Build history of the part. All positions in model axes, mm. A direction names the side the tool comes from. Round coordinates to 2 decimals unless told otherwise and drop trailing zeros. Loops run counter-clockwise (first coordinate to the right, second up) from the corner with the lowest first, then second, coordinate; pieces in that order, holes last.
from build123d import *

# Parameters (mm, degrees)
SKETCH_R        = 3.6
SKETCH_R_2      = 2.6
PAD_DEPTH       = 18
SKETCH001_R     = 3.6
POCKET_DEPTH    = 3
SKETCH002_W     = 40
SKETCH002_H     = 100
POCKET001_DEPTH = 8
SKETCH003_R     = 5.5
SKETCH003_R_2   = 4.5
POCKET002_DEPTH = 6
FILLET_R        = 6
FILLET001_R     = 6
SKETCH004_W     = 6.5
SKETCH004_H     = 33
POCKET003_DEPTH = 4
SKETCH005_R     = 2.1
POCKET004_DEPTH = 10
FILLET002_R     = 3.75


with BuildPart() as part:
    # Sketch → Pad (new body)
    with BuildSketch(Plane.XY):
        Polygon((-38.5, 0), (-38.5, 10), (19, 40), (38.5, 40), (38.5, 0), (38.5, -40), (19, -40), (-38.5, -10), align=None)
        with Locations((-28.5, 0)):
            Circle(SKETCH_R, mode=Mode.SUBTRACT)
        with Locations((28.5, -30)):
            Circle(SKETCH_R_2, mode=Mode.SUBTRACT)
        with Locations((28.5, 30)):
            Circle(SKETCH_R_2, mode=Mode.SUBTRACT)
    extrude(amount=PAD_DEPTH)

    # Sketch001 (on Face3 of Pad) → Pocket (cut)
    with BuildSketch(Plane(origin=(0, 0, 0), x_dir=(1, 0, 0), z_dir=(0, 0, -1))):
        with Locations((-28.5, 0)):
            Circle(SKETCH001_R)
    extrude(amount=-POCKET_DEPTH, mode=Mode.SUBTRACT)

    # Sketch002 (on Face3 of Pocket) → Pocket001 (cut)
    with BuildSketch(Plane(origin=(0, 0, 0), x_dir=(1, 0, 0), z_dir=(0, 0, -1))):
        Rectangle(SKETCH002_W, SKETCH002_H)
    extrude(amount=-POCKET001_DEPTH, mode=Mode.SUBTRACT)

    # Sketch003 (on Face6 of Pocket001) → Pocket002 (cut)
    with BuildSketch(Plane.XY.offset(18)):
        with Locations((-28.5, 0)):
            Circle(SKETCH003_R)
        with Locations((28.5, 30)):
            Circle(SKETCH003_R_2)
        with Locations((28.5, -30)):
            Circle(SKETCH003_R_2)
    extrude(amount=-POCKET002_DEPTH, mode=Mode.SUBTRACT)

    # Fillet
    fillet_edges = [part.edges().sort_by_distance(p)[0] for p in [
        (20, -40, 4),
        (20, 40, 4),
        (-20, -19.652174, 4),
        (-20, 19.652174, 4),
    ]]
    fillet(fillet_edges, radius=FILLET_R)

    # Fillet001
    fillet001_edges = [part.edges().sort_by_distance(p)[0] for p in [
        (-38.5, 10, 9),
        (-38.5, -10, 9),
        (19, 40, 13),
        (38.5, 40, 9),
        (38.5, -40, 9),
        (19, -40, 13),
    ]]
    fillet(fillet001_edges, radius=FILLET001_R)

    # Sketch004 (on Face5 of Fillet001) → Pocket003 (cut)
    with BuildSketch(Plane.XY.offset(18)):
        with Locations((0, -18.5)):
            Rectangle(SKETCH004_W, SKETCH004_H)
        with Locations((0, 18.5)):
            Rectangle(SKETCH004_W, SKETCH004_H)
    extrude(amount=-POCKET003_DEPTH, mode=Mode.SUBTRACT)

    # Sketch005 (on Face6 of Pocket003) → Pocket004 (cut)
    with BuildSketch(Plane.XY.offset(18)):
        with Locations((-15, 0)):
            Circle(SKETCH005_R)
        with Locations((15, -30)):
            Circle(SKETCH005_R)
        with Locations((15, 30)):
            Circle(SKETCH005_R)
    extrude(amount=-POCKET004_DEPTH, mode=Mode.SUBTRACT)

    # Fillet002
    fillet002_edges = [part.edges().sort_by_distance(p)[0] for p in [
        (0, -2, 14),
        (0, 2, 14),
    ]]
    fillet(fillet002_edges, radius=FILLET002_R)


solid = part.part
(1) Slice it at B-B on x = 28.5. List the corners of the cut face in (y, z), plus the area to 3 significant figures.
Responses:
outline: (-40, 0) - (-32.6, 0) - (-32.6, 12) - (-34.5, 12) - (-34.5, 18) - (-40, 18) - close; (-27.4, 0) - (27.4, 0) - (27.4, 12) - (25.5, 12) - (25.5, 18) - (-25.5, 18) - (-25.5, 12) - (-27.4, 12) - close; (32.6, 0) - (40, 0) - (40, 18) - (34.5, 18) - (34.5, 12) - (32.6, 12) - close
area: 1,210 mm2
(2) Pull direction X, two halves, no side cores. Call faces 1 (the face through (-9.16, 25.31, 12.87)), 2 (the face through (36.789, 38.196, 9.126)), 3 (the face through (0, 19, 14)): +X half, -X half, draft (parallel to the pull), parting line (faces both ways), or undercut.
Responses:
face 1: -X half
face 2: +X half
face 3: undercut
(3) Which spindle directions (+Z, -Z, +X, -X, +Y, -Y) get a long thin tool onto all of the face, cutting with end or side? Do faces 4 (the face through (-3.25, -15, 16)), 5 (the face through (20, 0, 4)), 6 (the face through (-27, -4, 12)), 7 (the face through (-22.964, 14.929, 3.944)), 8 (the face through (-3.25, 15, 16)). Say none if no direction does.
Responses:
face 4: +Z, -Y
face 5: -Z, +Y, -Y
face 6: +Z
face 7: -Z, +Y
face 8: +Z, +Y
(4) Slice it at A-A on z = 5. List the corners of the cut face in (x, y).
Responses:
outline: (-38.5, -6.36) arc R6 ccw to (-35.28, -11.68) - (-28.78, -15.07) arc R6 ccw to (-20, -9.75) - (-20, 9.75) arc R6 ccw to (-28.78, 15.07) - (-35.28, 11.68) arc R6 ccw to (-38.5, 6.36) - close; (20, -34) arc R6 ccw to (26, -40) - (32.5, -40) arc R6 ccw to (38.5, -34) - (38.5, 34) arc R6 ccw to (32.5, 40) - (26, 40) arc R6 ccw to (20, 34) - close; hole circle Ø7.2 at (-28.5, 0); hole circle Ø5.2 at (28.5, -30); hole circle Ø5.2 at (28.5, 30)
(5) Slice it at D-D on x = -15. List the corners of the cut face in (y, z), plus the area to 3 significant figures.
Responses:
outline: (-22.26, 8) - (-2.1, 8) - (-2.1, 18) - (-22.26, 18) - close; (2.1, 8) - (22.26, 8) - (22.26, 18) - (2.1, 18) - close
area: 403 mm2
(6) Probe line 1 (Y direction, x = 28.5, z = 8); line 2 (Y direction, x = 15, z = 15); line 3 (X direction, y = 15.5, z = 17). List the from-to ranges inside material, lowest first.
Responses:
line 1: y = -40 to -32.6, -27.4 to 27.4, 32.6 to 40
line 2: y = -37.91 to -32.1, -27.9 to 27.9, 32.1 to 37.91
line 3: x = -27.96 to -3.25, 3.25 to 38.5
(7) Slice it at C-C on z = 9. List the corners of the cut face in (x, y).
Responses:
outline: (-38.5, -6.36) arc R6 ccw to (-35.28, -11.68) - (17.7, -39.32) arc R6 ccw to (20.47, -40) - (32.5, -40) arc R6 ccw to (38.5, -34) - (38.5, 34) arc R6 ccw to (32.5, 40) - (20.47, 40) arc R6 ccw to (17.7, 39.32) - (-35.28, 11.68) arc R6 ccw to (-38.5, 6.36) - close; hole circle Ø7.2 at (-28.5, 0); hole circle Ø4.2 at (-15, 0); hole circle Ø4.2 at (15, -30); hole circle Ø4.2 at (15, 30); hole circle Ø5.2 at (28.5, -30); hole circle Ø5.2 at (28.5, 30)
(8) Pin check, flat tips, straight feed: P1, Ø8, axis at x = 28.5, y = 30, coming from the -Z side; P2, Ø6.5, axis at x = -15, y = 0, coming from the -Z side; P3, Ø3, axis at x = 0.5, y = 22.5, coming from the +Z side; P4, Ø8, axis at x = -7, z = 7, coming from the +Y side. Stop position of each tip, or through.
Responses:
P1: stops at z = 0
P2: stops at z = 8
P3: stops at z = 14
P4: stops at y = 28.46
